The model under review builds one solid part; all positions refer to its coordinate system, in mm. A direction names the side the tool comes from. Round coordinates to 2 decimals unless told otherwise and drop trailing zeros. Write each loop counter-clockwise with the first axis right and the second up, starting at its lowest first coordinate (ties: lowest second). Pieces come first, ordered by that corner, then holes. Notation, with made-up numbers: (-16, 9) -> (34, 9) arc R18 cw to (34, 36) -> close; hole circle Ø5 at (42.25, -9). An arc over 180 degrees is marked (long way). Answer as a JSON object with one key per item and string values. Group by question number.
1) We need section B-B, the plane y = 58.5. Write out the cut boundary in (x, z).
2) Machinability: for faces 4 (the flat face through (20, 52, -8)), 5 (the flat face through (-10, 68, -8)), 6 (the flat face through (-20, 53, -8)), which of the approach directions +Z, -Z, +X, -X, +Y, -Y give a long, thin tool a straight path to every point of the face, cutting with its end or side? Answer none if there is none.
3) We need section A-A, the plane x = 0. Write out the cut boundary in (y, z), then the cut area to 3 significant figures.
4) Insertion check: pin 1 Ø1 at (x, z) = (12.5, 1) entering from -Y; pin 2 Ø6 at (x, y) = (-6, 41) entering from -Z; pin 3 Ø5 at (y, z) = (77.5, 4) entering from -X; pin 4 Ø8 at (y, z) = (61.5, -8) entering from +X. Each pin has a flat end and moves straight along its axis. Give the tip position at first contact, or say it passes through.
5) We need section D-D, the plane y = 0. Write out the cut boundary in (x, z).
6) Mouldability with a two-part tool opening along X and no side actions: class faces 1 (the cylindrical face through (13.44, -21.08, -8.25)), 2 (the flat face through (10, 67, -8)), 3 (the flat face through (-5.9, 11.5, -25.5)) as pulls with the +X half, pulls with the -X half, needs draft (parallel to the pull), parting line crosses it, or undercut.
7) We need section C-C, the plane z = 3.5. Write out the cut boundary in (x, y), then the cut area to 3 significant figures.
8) To check wall thickness, follow probe 1 along Y at (x, z) = (0, -15); probe 2 along X at (y, z) = (85, -1); probe 3 along Y at (x, z) = (-2, -11). State the ranges of each line that lie inside material, in increasing order. Write a range as [from, to].
Autodesk Inventor part; units mm, degrees
ref_plane "YZ Plane" through (0, 0, 0) normal (1, 0, 0) x (0, 1, 0)
ref_plane "XZ Plane" through (0, 0, 0) normal (0, 1, 0) x (-1, 0, 0)
ref_plane "XY Plane" through (0, 0, 0) normal (0, 0, 1) x (1, 0, 0)
sketch "Náčrt1" plane through (0, 0, 0) normal (0, 0, 1) x (1, 0, 0)
  circle A0 centre (0, 0) radius 25
  dimension "d0" = 50
extrude "Vysunutí1" add sketch "Náčrt1" against normal blind 25.5
sketch "Náčrt2" plane through (0, 0, 0) normal (0, 0, 1) x (1, 0, 0)
  circle A0 centre (0, 0) radius 12.5
  dimension "d3" = 25
extrude "Vysunutí2" cut sketch "Náčrt2" against normal blind 35
sketch "Náčrt3" plane through (0, 0, 0) normal (0, 0, 1) x (1, 0, 0)
  circle A0 centre (0, 0) radius 25
  line L0 (20, 15) -> (20, 90)
  arc A1 (20, 90) -> (-20, 90) centre (0, 90) ccw
  line L1 (-20, 90) -> (-20, 15)
  arc A2 (10, 90) -> (-10, 90) centre (0, 90) ccw
  line L2 (-10, 90) -> (-10, 45)
  arc A3 (-10, 45) -> (10, 45) centre (0, 45) ccw
  line L3 (10, 45) -> (10, 90)
  arc A4 (20, 15) -> (-20, 15) centre (0, 0) ccw
  dimension "d7" = 90
  dimension "d8" = 40
  dimension "d9" = 20
  dimension "d10" = 20
  dimension "d11" = 10
  dimension "d12" = 45
extrude "Vysunutí3" add sketch "Náčrt3" against normal blind 16 contours A0 L1 A1 L0
sketch "Náčrt4" plane through (0, 0, 0) normal (0, 0, 1) x (1, 0, 0)
  circle A0 centre (0, 0) radius 25
  circle A1 centre (0, 0) radius 25
  circle A2 centre (0, 0) radius 12.5
extrude "Vysunutí4" add sketch "Náčrt4" along normal blind 9.5
fillet "Zaoblení1" radius 5 1 edges at (0, 25, 0)
fillet "Zaoblení2" radius 5 1 edges at (0, 25, -16)
properties part number "13"
Here are the results:
{
 "1": {"outline": "(-20, -16) -> (-10, -16) -> (-10, 0) -> (-20, 0) -> close; (10, -16) -> (20, -16) -> (20, 0) -> (10, 0) -> close"},
 "2": {"face 4": "+Z, -Z, +X, +Y", "face 5": "+Z, -Z", "face 6": "+Z, -Z, -X, +Y"},
 "3": {"outline": "(-25, -25.5) -> (-12.5, -25.5) -> (-12.5, 9.5) -> (-25, 9.5) -> close; (12.5, -25.5) -> (25, -25.5) -> (25, -21) arc R5 cw to (30, -16) -> (35, -16) -> (35, 0) -> (30, 0) arc R5 cw to (25, 5) -> (25, 9.5) -> (12.5, 9.5) -> close; (100, -16) -> (110, -16) -> (110, 0) -> (100, 0) -> close", "area": "1,210 mm^2"},
 "4": {"pin 1": "stops at y = -21.93", "pin 2": "stops at z = -16", "pin 3": "passes through", "pin 4": "stops at x = 20"},
 "5": {"outline": "(-25, -25.5) -> (-12.5, -25.5) -> (-12.5, 9.5) -> (-25, 9.5) -> close; (12.5, -25.5) -> (25, -25.5) -> (25, 9.5) -> (12.5, 9.5) -> close"},
 "6": {"face 1": "parting line crosses it", "face 2": "undercut", "face 3": "needs draft"},
 "7": {"outline": "(-20, 15) arc R25 ccw (long way) to (20, 15) -> (20, 15.38) arc R25.23 ccw to (-20, 15.38) -> close; hole circle Ø25 at (0, 0)", "area": "1,480 mm^2"},
 "8": {"probe 1": "y = [-25, -12.5], [12.5, 35], [100, 110]", "probe 2": "x = [-20, -10], [10, 20]", "probe 3": "y = [-24.92, -12.34], [12.34, 35.2], [99.8, 109.9]"}
}
